CAD build for the part. Positions are in the model's coordinates, mm. A direction names the side the tool comes from. Coordinates: 2 decimals unless noted, no trailing zeros. Order: outer loops, then holes, each group sorted by start corner. A loop starts at its lowest first (then second) coordinate and runs counter-clockwise, first axis right, second up. Notation, with made-up numbers: (29, -13) - (63, -13) arc R18 cw to (63, 6) - close; hole circle Ø7 at (-37.75, 64). An arc over 180 degrees is marked (long way). Write each question's results on one line, items separated by ' | '. Start each with the question number.
Q1. Which spindle directions (+Z, -Z, +X, -X, +Y, -Y) get a long thin tool onto all of the face, cutting with end or side? Do faces 1 (the flat face through (107.5, 37, 1)), 2 (the cylindrical face through (107.298, 2.521, -58.278)), 3 (the cylindrical face through (105.979, 13.304, -0.43)). Say none if no direction does.
Q2. Band-saw the part on B-B, the plane z = -26.5. Write the cut outline in (x, y), then the cut area to 3 significant figures.
Q3. Wall check: probe 1 along Y at (x, z) = (105.8, 0); probe 2 along X at (y, z) = (0.45, 61.5); probe 3 along X at (y, z) = (44, -43). Give the ranges that are in metal, low to high.
Q4. Band-saw the part on D-D, the plane z = 44.5. Write the cut outline in (x, y), then the cut area to 3 significant figures.
Q5. Band-saw the part on C-C, the plane x = -82.5. Write the cut outline in (y, z).
Q6. Pin check, flat tips, straight feed: P1, Ø6, axis at y = 51.31, z = 0, coming from the +X side; P2, Ø5, axis at y = 27.5, z = -12.5, coming from the -X side; P3, Ø2.5, axis at y = 59, z = 13, coming from the -X side. Stop position of each tip, or through.
Q7. Pull direction Z, two halves, no side cores. Call faces 4 (the flat face through (1, 4, 60)), 5 (the flat face through (-109, 1, 61)), 6 (the flat face through (-104.5, 28, 1)), 7 (the cylindrical face through (-115.73, 1.97, 65.64)): released by +Z, released by -Z, zero draft, split by the parting line, or undercut.
Q8. Band-saw the part on A-A, the plane x = 84.5. Write the cut outline in (y, z).
```python
from build123d import *

# Parameters (mm, degrees)
BOSS_EXTRU_1_DEPTH                                 = 60
COQUE1_T                                           = -3
BOSS_EXTRU_2_OUTLINE_W                             = 196
BOSS_EXTRU_2_OUTLINE_H                             = 96.5
BOSS_EXTRU_2_DEPTH                                 = 10
ESQUISSE3_W                                        = 71
ESQUISSE3_H                                        = 39.5
ESQUISSE3_W_2                                      = 11.5
ESQUISSE3_H_2                                      = 4
ENL_V_MAT_EXTRU_1_DEPTH                            = 3
ESQUISSE3_4_W                                      = 25.2
ESQUISSE3_4_H                                      = 27.8
ENL_V_MAT_EXTRU_2_DEPTH                            = 2
ESQUISSE5_W                                        = 184
ESQUISSE5_H                                        = 84.5
ENL_V_MAT_EXTRU_3_DEPTH                            = 3
ENL_V_MAT_EXTRU_4_REACH                            = 235.305
ESQUISSE8_W                                        = 30
ESQUISSE8_H                                        = 15
ESQUISSE9_W                                        = 209
ESQUISSE9_H                                        = 109
BOSS_EXTRU_4_DEPTH                                 = 4
CHAMBRAGE_POUR_VIS_T_TE_HEXAGONALE_M41_D           = 4.5
CHAMBRAGE_POUR_VIS_T_TE_HEXAGONALE_M41_CBORE_D     = 10.59
CHAMBRAGE_POUR_VIS_T_TE_HEXAGONALE_M41_CBORE_DEPTH = 3
ENL_V_MAT_EXTRU_5_DEPTH                            = 3
D_GAGEMENT_M61_D                                   = 6.6
D_GAGEMENT_M61_DEPTH                               = 3


# Read off the part's stored shape, not the designer's step: Boss.-Extru.2
with BuildPart() as part:
    # Esquisse1 → Boss.-Extru.1 (new body)
    with BuildSketch(Plane(origin=(0, 0, 0), x_dir=(1, 0, 0), z_dir=(0, 1, 0))):
        with BuildLine():
            Line((-103.5, 57.5), (103.5, 57.5))
            ThreePointArc((103.5, 57.5), (106.328427125, 56.328427125), (107.5, 53.5))
            Line((107.5, 53.5), (107.5, -53.5))
            ThreePointArc((107.5, -53.5), (106.328427125, -56.328427125), (103.5, -57.5))
            Line((103.5, -57.5), (-103.5, -57.5))
            ThreePointArc((-103.5, -57.5), (-106.328427125, -56.328427125), (-107.5, -53.5))
            Line((-107.5, -53.5), (-107.5, 53.5))
            ThreePointArc((-107.5, 53.5), (-106.328427125, 56.328427125), (-103.5, 57.5))
        make_face()
    extrude(amount=BOSS_EXTRU_1_DEPTH)

    # Coque1
    coque1_openings = [part.faces().sort_by_distance(p)[0] for p in [
        (0, 0, 0),
    ]]
    offset(amount=COQUE1_T, openings=coque1_openings, kind=Kind.INTERSECTION)

    # Boss.-Extru.2 outline → Boss.-Extru.2 (add)
    with BuildSketch(Plane(origin=(0, 60, 0), x_dir=(1, 0, 0), z_dir=(0, 1, 0))):
        with BuildLine():
            ThreePointArc((-103.5, 57.5), (-106.328427125, 56.328427125), (-107.5, 53.5))
            Line((-107.5, 53.5), (-107.5, -53.5))
            ThreePointArc((-107.5, -53.5), (-106.328427125, -56.328427125), (-103.5, -57.5))
            Line((-103.5, -57.5), (103.5, -57.5))
            ThreePointArc((103.5, -57.5), (106.328427125, -56.328427125), (107.5, -53.5))
            Line((107.5, -53.5), (107.5, 53.5))
            ThreePointArc((107.5, 53.5), (106.328427125, 56.328427125), (103.5, 57.5))
            Line((103.5, 57.5), (-103.5, 57.5))
        make_face()
        Rectangle(BOSS_EXTRU_2_OUTLINE_W, BOSS_EXTRU_2_OUTLINE_H, mode=Mode.SUBTRACT)
    extrude(amount=BOSS_EXTRU_2_DEPTH)

    # Esquisse3 → Enlèv. mat.-Extru.1 (cut)
    with BuildSketch(Plane(origin=(0, 0, -57.5), x_dir=(-1, 0, 0), z_dir=(0, 0, -1))):
        with Locations((-55, 35)):
            Rectangle(ESQUISSE3_W, ESQUISSE3_H)
        with Locations((8.072937115, 46.188484734)):
            Rectangle(ESQUISSE3_W_2, ESQUISSE3_H_2)
        with BuildLine():
            ThreePointArc((38.117871013, 28.332487519), (39.61171058, 29.660770737), (40.166695713, 31.581157276))
            ThreePointArc((40.166695713, 31.581157276), (40.163949212, 31.721753371), (40.155713901, 31.862134939))
            ThreePointArc((40.155713901, 31.862134939), (39.251374465, 33.131157276), (38.604538601, 34.54884937))
            ThreePointArc((38.604538601, 34.54884937), (36.566695713, 35.181157276), (34.528852825, 34.54884937))
            ThreePointArc((34.528852825, 34.54884937), (33.882016961, 33.131157276), (32.977677525, 31.862134939))
            ThreePointArc((32.977677525, 31.862134939), (33.449004259, 29.781157276), (35.015520413, 28.332487519))
            ThreePointArc((35.015520413, 28.332487519), (36.566695713, 28.481157276), (38.117871013, 28.332487519))
        make_face()
        with BuildLine():
            ThreePointArc((-1.233296382, 45.916330985), (-1.820845102, 46.388484734), (-1.935967883, 47.133393726))
            ThreePointArc((-1.935967883, 47.133393726), (-2.427062885, 47.238484734), (-2.918157886, 47.133393726))
            ThreePointArc((-2.918157886, 47.133393726), (-3.033280667, 46.388484734), (-3.620829387, 45.916330985))
            ThreePointArc((-3.620829387, 45.916330985), (-3.466293369, 45.438484734), (-3.129734385, 45.065729492))
            ThreePointArc((-3.129734385, 45.065729492), (-2.427062885, 45.338484734), (-1.724391384, 45.065729492))
            ThreePointArc((-1.724391384, 45.065729492), (-1.3878324, 45.438484734), (-1.233296382, 45.916330985))
        make_face()
        with BuildLine():
            ThreePointArc((17.379170613, 45.916330985), (17.533706631, 45.438484734), (17.870265615, 45.065729492))
            ThreePointArc((17.870265615, 45.065729492), (18.572937115, 45.338484734), (19.275608616, 45.065729492))
            ThreePointArc((19.275608616, 45.065729492), (19.6121676, 45.438484734), (19.766703618, 45.916330985))
            ThreePointArc((19.766703618, 45.916330985), (19.179154898, 46.388484734), (19.064032117, 47.133393726))
            ThreePointArc((19.064032117, 47.133393726), (18.572937115, 47.238484734), (18.081842114, 47.133393726))
            ThreePointArc((18.081842114, 47.133393726), (17.966719333, 46.388484734), (17.379170613, 45.916330985))
        make_face()
        with BuildLine():
            ThreePointArc((-1.233296382, 22.416330985), (-1.820845102, 22.888484734), (-1.935967883, 23.633393726))
            ThreePointArc((-1.935967883, 23.633393726), (-2.427062885, 23.738484734), (-2.918157886, 23.633393726))
            ThreePointArc((-2.918157886, 23.633393726), (-3.033280667, 22.888484734), (-3.620829387, 22.416330985))
            ThreePointArc((-3.620829387, 22.416330985), (-3.466293369, 21.938484734), (-3.129734385, 21.565729492))
            ThreePointArc((-3.129734385, 21.565729492), (-2.427062885, 21.838484734), (-1.724391384, 21.565729492))
            ThreePointArc((-1.724391384, 21.565729492), (-1.3878324, 21.938484734), (-1.233296382, 22.416330985))
        make_face()
        with BuildLine():
            ThreePointArc((19.766703618, 22.416330985), (19.179154898, 22.888484734), (19.064032117, 23.633393726))
            ThreePointArc((19.064032117, 23.633393726), (18.572937115, 23.738484734), (18.081842114, 23.633393726))
            ThreePointArc((18.081842114, 23.633393726), (17.966719333, 22.888484734), (17.379170613, 22.416330985))
            ThreePointArc((17.379170613, 22.416330985), (17.533706631, 21.938484734), (17.870265615, 21.565729492))
            ThreePointArc((17.870265615, 21.565729492), (18.572937115, 21.838484734), (19.275608616, 21.565729492))
            ThreePointArc((19.275608616, 21.565729492), (19.6121676, 21.938484734), (19.766703618, 22.416330985))
        make_face()
    extrude(amount=-ENL_V_MAT_EXTRU_1_DEPTH, mode=Mode.SUBTRACT)

    # Esquisse3<4> → Enlèv. mat.-Extru.2 (cut)
    with BuildSketch(Plane(origin=(0, 0, -57.5), x_dir=(-1, 0, 0), z_dir=(0, 0, -1))):
        with Locations((8.072937115, 34.288484734)):
            Rectangle(ESQUISSE3_4_W, ESQUISSE3_4_H)
    extrude(amount=-ENL_V_MAT_EXTRU_2_DEPTH, mode=Mode.SUBTRACT)

    # Esquisse5 → Enlèv. mat.-Extru.3 (cut)
    with BuildSketch(Plane(origin=(0, 60, 0), x_dir=(1, 0, 0), z_dir=(0, 1, 0))):
        Rectangle(ESQUISSE5_W, ESQUISSE5_H)
    extrude(amount=-ENL_V_MAT_EXTRU_3_DEPTH, mode=Mode.SUBTRACT)

    # Esquisse8 → Enlèv. mat.-Extru.4 (cut, up to next)
    with BuildSketch(Plane.ZY.offset(107.5), mode=Mode.PRIVATE) as enl_v_mat_extru_4_sk1:
        with Locations((-18.5, 27.5)):
            Rectangle(ESQUISSE8_W, ESQUISSE8_H)
    enl_v_mat_extru_4_tool1 = extrude(enl_v_mat_extru_4_sk1.sketch, amount=-ENL_V_MAT_EXTRU_4_REACH, mode=Mode.PRIVATE) & part.part
    add(enl_v_mat_extru_4_tool1.solids().sort_by_distance((-107.5, 27.5, -18.5))[0], mode=Mode.SUBTRACT)

    # Esquisse9 → Boss.-Extru.4 (add)
    with BuildSketch(Plane.XZ):
        with BuildLine():
            Line((111.3, -67.5), (-111.3, -67.5))
            ThreePointArc((-111.3, -67.5), (-115.684062043, -65.684062043), (-117.5, -61.3))
            Line((-117.5, -61.3), (-117.5, 61.3))
            ThreePointArc((-117.5, 61.3), (-115.684062043, 65.684062043), (-111.3, 67.5))
            Line((-111.3, 67.5), (111.3, 67.5))
            ThreePointArc((111.3, 67.5), (115.684062043, 65.684062043), (117.5, 61.3))
            Line((117.5, 61.3), (117.5, -61.3))
            ThreePointArc((117.5, -61.3), (115.684062043, -65.684062043), (111.3, -67.5))
        make_face()
        Rectangle(ESQUISSE9_W, ESQUISSE9_H, mode=Mode.SUBTRACT)
    extrude(amount=-BOSS_EXTRU_4_DEPTH)

    # Chambrage pour vis à tête hexagonale M41 (through all)
    with Locations(Plane(origin=(0, 4, 0), x_dir=(1, 0, 0), z_dir=(0, 1, 0))):
        with Locations((-111.5, 61.5), (111.5, 61.5), (111.5, -61.5), (-111.5, -61.5)):
            CounterBoreHole(CHAMBRAGE_POUR_VIS_T_TE_HEXAGONALE_M41_D / 2, CHAMBRAGE_POUR_VIS_T_TE_HEXAGONALE_M41_CBORE_D / 2, CHAMBRAGE_POUR_VIS_T_TE_HEXAGONALE_M41_CBORE_DEPTH)

    # Esquisse13 → Enlèv. mat.-Extru.5 (cut)
    with BuildSketch(Plane(origin=(107.5, 0, 0), x_dir=(0, 0, -1), z_dir=(1, 0, 0))):
        with BuildLine():
            ThreePointArc((8.193649051, 24.74946516), (7.299038106, 25.666509594), (6.952159802, 26.899787616))
            ThreePointArc((6.952159802, 26.899787616), (6, 27.116509594), (5.047840198, 26.899787616))
            ThreePointArc((5.047840198, 26.899787616), (4.700961894, 25.666509594), (3.806350949, 24.74946516))
            ThreePointArc((3.806350949, 24.74946516), (4.094744112, 23.816509594), (4.758510751, 23.100276006))
            ThreePointArc((4.758510751, 23.100276006), (6, 23.416509594), (7.241489249, 23.100276006))
            ThreePointArc((7.241489249, 23.100276006), (7.905255888, 23.816509594), (8.193649051, 24.74946516))
        make_face()
        with BuildLine():
            ThreePointArc((51.952159802, 26.899787616), (51, 27.116509594), (50.047840198, 26.899787616))
            ThreePointArc((50.047840198, 26.899787616), (49.700961894, 25.666509594), (48.806350949, 24.74946516))
            ThreePointArc((48.806350949, 24.74946516), (49.094744112, 23.816509594), (49.758510751, 23.100276006))
            ThreePointArc((49.758510751, 23.100276006), (51, 23.416509594), (52.241489249, 23.100276006))
            ThreePointArc((52.241489249, 23.100276006), (52.905255888, 23.816509594), (53.193649051, 24.74946516))
            ThreePointArc((53.193649051, 24.74946516), (52.299038106, 25.666509594), (51.952159802, 26.899787616))
        make_face()
        with BuildLine():
            ThreePointArc((-48.806350949, 24.74946516), (-49.700961894, 25.666509594), (-50.047840198, 26.899787616))
            ThreePointArc((-50.047840198, 26.899787616), (-51, 27.116509594), (-51.952159802, 26.899787616))
            ThreePointArc((-51.952159802, 26.899787616), (-52.299038106, 25.666509594), (-53.193649051, 24.74946516))
            ThreePointArc((-53.193649051, 24.74946516), (-52.905255888, 23.816509594), (-52.241489249, 23.100276006))
            ThreePointArc((-52.241489249, 23.100276006), (-51, 23.416509594), (-49.758510751, 23.100276006))
            ThreePointArc((-49.758510751, 23.100276006), (-49.094744112, 23.816509594), (-48.806350949, 24.74946516))
        make_face()
        with BuildLine():
            ThreePointArc((-5.047840198, 26.899787616), (-6, 27.116509594), (-6.952159802, 26.899787616))
            ThreePointArc((-6.952159802, 26.899787616), (-7.299038106, 25.666509594), (-8.193649051, 24.74946516))
            ThreePointArc((-8.193649051, 24.74946516), (-7.905255888, 23.816509594), (-7.241489249, 23.100276006))
            ThreePointArc((-7.241489249, 23.100276006), (-6, 23.416509594), (-4.758510751, 23.100276006))
            ThreePointArc((-4.758510751, 23.100276006), (-4.094744112, 23.816509594), (-3.806350949, 24.74946516))
            ThreePointArc((-3.806350949, 24.74946516), (-4.700961894, 25.666509594), (-5.047840198, 26.899787616))
        make_face()
    extrude(amount=-ENL_V_MAT_EXTRU_5_DEPTH, mode=Mode.SUBTRACT)

    # Dégagement M61
    with Locations(Plane(origin=(107.5, 0, 0), x_dir=(0, 0, -1), z_dir=(1, 0, 0))):
        with Locations((0, 51.309466908), (0, 10.031656552)):
            Hole(D_GAGEMENT_M61_D / 2, depth=D_GAGEMENT_M61_DEPTH)


solid = part.part
```
Results below:
1) face 1: +Z, -Z, +X, +Y | face 2: +Y | face 3: +X
2) outline: (-117.5, 0) - (-104.5, 0) - (-104.5, 20) - (-107.5, 20) - (-107.5, 4) - (-117.5, 4) - close; (-107.5, 35) - (-104.5, 35) - (-104.5, 57) - (-92, 57) - (-92, 60) - (-98, 60) - (-98, 70) - (-107.5, 70) - close; (92, 57) - (104.5, 57) - (104.5, 0) - (117.5, 0) - (117.5, 4) - (107.5, 4) - (107.5, 70) - (98, 70) - (98, 60) - (92, 60) - close | area: 660 mm²
3) probe 1: y = 0 to 6.73, 13.33 to 48.01, 54.61 to 70 | probe 2: x = -117.5 to -113.75, -109.25 to 109.25, 113.75 to 117.5 | probe 3: x = -107.5 to -104.5, 104.5 to 107.5
4) outline: (-117.5, 0) - (-104.5, 0) - (-104.5, 57) - (104.5, 57) - (104.5, 0) - (117.5, 0) - (117.5, 4) - (107.5, 4) - (107.5, 70) - (98, 70) - (98, 60) - (-98, 60) - (-98, 70) - (-107.5, 70) - (-107.5, 4) - (-117.5, 4) - close | area: 1,260 mm²
5) outline: (0, -67.5) - (4, -67.5) - (4, -57.5) - (70, -57.5) - (70, -48.25) - (60, -48.25) - (60, -42.25) - (57, -42.25) - (57, -54.5) - (0, -54.5) - close; (0, 54.5) - (57, 54.5) - (57, 42.25) - (60, 42.25) - (60, 48.25) - (70, 48.25) - (70, 57.5) - (4, 57.5) - (4, 67.5) - (0, 67.5) - close
6) P1: stops at x = -104.5 | P2: stops at x = 104.5 | P3: stops at x = -107.5
7) face 4: zero draft | face 5: undercut | face 6: undercut | face 7: released by +Z
8) outline: (0, -67.5) - (4, -67.5) - (4, -57.5) - (15.25, -57.5) - (15.25, -54.5) - (0, -54.5) - close; (0, 54.5) - (57, 54.5) - (57, 42.25) - (60, 42.25) - (60, 48.25) - (70, 48.25) - (70, 57.5) - (4, 57.5) - (4, 67.5) - (0, 67.5) - close; (54.75, -57.5) - (70, -57.5) - (70, -48.25) - (60, -48.25) - (60, -42.25) - (57, -42.25) - (57, -54.5) - (54.75, -54.5) - close
